Verification items for the finished model (mm, model axes). A direction names the side the tool comes from. Coordinates: 2 decimals unless noted, no trailing zeros. Write each loop counter-clockwise with the first axis right and the second up, starting at its lowest first coordinate (ties: lowest second). Pieces come first, ordered by that corner, then holes. Notation, with made-up numbers: (27.5, 35.25) -> (47.5, 35.25) arc R19 cw to (47.5, 72.25) -> close; hole circle Ø5 at (36, 45). An arc over 180 degrees is marked (long way). Use CSV: the item, a comma, the result in double quotes.
```python
from build123d import *

# Parameters (mm, degrees)
SKETCH1_R             = 2.5
BOSS_EXTRUDE1_DEPTH   = 3
SKETCH1_W             = 30
SKETCH1_H             = 70
BOSS_EXTRUDE1_2_DEPTH = 3
SKETCH3_W             = 30
SKETCH3_H             = 10
BOSS_EXTRUDE2_DEPTH   = 8
SKETCH4_W             = 3
SKETCH4_H             = 150
BOSS_EXTRUDE4_DEPTH   = 23
SKETCH5_R             = 3
CUT_EXTRUDE1_DEPTH    = 23
SKETCH6_W             = 26
SKETCH6_H             = 3
BOSS_EXTRUDE5_DEPTH   = 3
FILLET1_R             = 10
SKETCH7_W             = 36.729037069
SKETCH7_H             = 60
CUT_EXTRUDE2_DEPTH    = 3
FILLET2_R             = 10


with BuildPart() as part:
    # Sketch1 → Boss-Extrude1 (new body)
    with BuildSketch(Plane.XY):
        Polygon((30, 150), (0, 150), (-10, 150), (-10, 120), (0, 120), (0, 80), (30, 80), (30, 120), align=None)
        with Locations((0, 130)):
            Circle(SKETCH1_R, mode=Mode.SUBTRACT)
    extrude(amount=-BOSS_EXTRUDE1_DEPTH)



with BuildPart() as body_2:
    # Sketch1 → Boss-Extrude1 2 (new body)
    with BuildSketch(Plane.XY):
        with Locations((15, 35)):
            Rectangle(SKETCH1_W, SKETCH1_H)
        with Locations((15, 20)):
            Circle(SKETCH1_R, mode=Mode.SUBTRACT)
    extrude(amount=-BOSS_EXTRUDE1_2_DEPTH)


with BuildPart() as part_1:
    add(part.part)

    add(body_2.part)  # Boss-Extrude2 merges body 2
    # Sketch3 → Boss-Extrude2 (add)
    with BuildSketch(Plane.XY):
        with Locations((15, 75)):
            Rectangle(SKETCH3_W, SKETCH3_H)
    extrude(amount=-BOSS_EXTRUDE2_DEPTH)

    # Sketch4 → Boss-Extrude4 (add)
    with BuildSketch(Plane.XY):
        with Locations((28.5, 75)):
            Rectangle(SKETCH4_W, SKETCH4_H)
    extrude(amount=BOSS_EXTRUDE4_DEPTH)

    # Sketch5 → Cut-Extrude1 (cut)
    with BuildSketch(Plane.ZY.offset(-27)):
        with Locations(Location((11.5, 75, 0), (0, 0, 270))):
            Circle(SKETCH5_R)
    extrude(amount=-CUT_EXTRUDE1_DEPTH, mode=Mode.SUBTRACT)

    # Sketch6 → Boss-Extrude5 (add)
    with BuildSketch(Plane(origin=(30, 0, 0), x_dir=(0, 0, -1), z_dir=(1, 0, 0))):
        with Locations((-10, 118.5)):
            Rectangle(SKETCH6_W, SKETCH6_H)
    extrude(amount=BOSS_EXTRUDE5_DEPTH)

    # Fillet1
    fillet1_edges = [part_1.edges().sort_by_distance(p)[0] for p in [
        (0, 0, -1.5),
        (28.5, 0, 23),
        (28.5, 150, 23),
        (-10, 120, -1.5),
        (-10, 150, -1.5),
    ]]
    fillet(fillet1_edges, radius=FILLET1_R - 0.0001)  # a hair under: the kernel refuses the full size

    # Sketch7 → Cut-Extrude2 (cut)
    with BuildSketch(Plane(origin=(30, 0, 0), x_dir=(0, 0, -1), z_dir=(1, 0, 0))):
        with Locations((-18.364518535, 30)):
            Rectangle(SKETCH7_W, SKETCH7_H)
    extrude(amount=-CUT_EXTRUDE2_DEPTH, mode=Mode.SUBTRACT)

    # Fillet2
    fillet2_edges = [part_1.edges().sort_by_distance(p)[0] for p in [
        (28.5, 60, 23),
    ]]
    fillet(fillet2_edges, radius=FILLET2_R)


solid = part_1.part
```
1) Cross-section at C-C (x = 23.5). Record the boundary of the cut face in (y, z), plus the area to 3 significant figures.
Return value:
outline,"(0, -3) -> (70, -3) -> (70, -8) -> (80, -8) -> (80, -3) -> (150, -3) -> (150, 0) -> (0, 0) -> close"
area,"500 mm2"
2) Set-up check for faces 4 (the flat face through (30, 135, 10)), 5 (the flat face through (15, 35, -3)), 6 (the flat face through (27, 104, 11)): record each of +Z, -Z, +X, -X, +Y, -Y from which the full face is reachable in a straight line by a thin tool's end or side.
Return value:
face 4,"+Z, -Z, +X, +Y"
face 5,"-Z, +X, -X, -Y"
face 6,"+Z, -X, +Y, -Y"
3) Cross-section at D-D (y = 75). Record the boundary of the cut face in (x, z), plus the area to 3 significant figures.
Return value:
outline,"(0, -8) -> (30, -8) -> (30, 8.5) -> (27, 8.5) -> (27, 0) -> (0, 0) -> close; (27, 14.5) -> (30, 14.5) -> (30, 23) -> (27, 23) -> close"
area,"291 mm2"
4) Gauge pin test, flat ends, axial feed: pin 1 (1.5 mm diameter, centred on x = 13, z = -4.5, fed in from +Y); pin 2 (9 mm diameter, centred on x = 9.5, y = 48.5, fed in from -Z); pin 3 (7 mm diameter, centred on y = 105.5, z = 16, fed in from -X); pin 4 (4 mm diameter, centred on x = 13.5, z = -4.5, fed in from -Y). Record the tip position at first contact, or that the pin passes through.
Return value:
pin 1,"y = 80"
pin 2,"z = -3"
pin 3,"x = 27"
pin 4,"y = 0"
5) Scan lines: L1, parallel to Z at x = 29.25, y = 75; L2, parallel to X at y = 130, z = -1.55; L3, parallel to Y at x = 15, z = -1.6. Record each from-to range of solid material in increasing order.
Return value:
L1,"-8 to 8.5, 14.5 to 23"
L2,"-10 to -2.5, 2.5 to 30"
L3,"0 to 17.5, 22.5 to 150"
6) Cross-section at B-B (z = 11.5). Record the boundary of the cut face in (x, y), plus the area to 3 significant figures.
Return value:
outline,"(27, 60) -> (30, 60) -> (30, 72) -> (27, 72) -> close; (27, 78) -> (30, 78) -> (30, 117) -> (33, 117) -> (33, 120) -> (30, 120) -> (30, 150) -> (27, 150) -> close"
area,"261 mm2"
7) Mould release check, pull along Y, two halves, no side actions. Record for faces 1 (the flat face through (11, 115, -3)), 2 (the flat face through (19.4, 150, -0.4)), 3 (the cylindrical face through (28.5, 77.4, 9.7)): released by +Y, released by -Y, zero draft, split by the parting line, or undercut.
Return value:
face 1,"zero draft"
face 2,"released by +Y"
face 3,"undercut"
8) Cross-section at A-A (y = 20). Record the boundary of the cut face in (x, z), plus the area to 3 significant figures.
Return value:
outline,"(0, -3) -> (12.5, -3) -> (12.5, 0) -> (0, 0) -> close; (17.5, -3) -> (30, -3) -> (30, 0) -> (17.5, 0) -> close"
area,"75.0 mm2"
